Autodesk Fusion 360 part; units mm, degrees
sketch "Sketch1" plane through (0, 0, 0) normal (0, 0, 1) x (1, 0, 0)
  line L0 (17, -17) -> (-17, -17) construction
  line L1 (-17, -17) -> (-17, 17) construction
  line L2 (-17, 17) -> (17, 17) construction
  line L3 (17, 17) -> (17, -17) construction
  line L4 (17, -17) -> (-17, 17) construction
  line L5 (-17, -17) -> (17, 17) construction
  circle A0 centre (17, -17) radius 3
  circle A1 centre (17, 17) radius 3
  circle A2 centre (-17, 17) radius 3
  circle A3 centre (-17, -17) radius 3
  line L6 (-19, -9.5) -> (19, -9.5) construction
  circle A4 centre (19, -9.5) radius 1.5
  circle A5 centre (-19, -9.5) radius 1.5
  circle A6 centre (0, 0) radius 26
  dimension "d1" = 34
  dimension "d2" = 34
  dimension "d3" = 6
  dimension "d4" = 6
  dimension "d5" = 6
  dimension "d6" = 6
  dimension "d7" = 38
  dimension "d8" = 7.5
  dimension "d9" = 3
  dimension "d10" = 3
  dimension "d11" = 52
extrude "Extrude1" add sketch "Sketch1" along normal blind 1.6 contours A0 A1 A2 A3 A6
sketch "Sketch2" plane through (0, 0, 1.6) normal (0, 0, 1) x (1, 0, 0)
  circle A0 centre (-19, -9.5) radius 1.5
  circle A1 centre (19, -9.5) radius 1.5
  line L0 (6, 19) -> (6, 15)
  line L1 (-6, 19) -> (6, 19)
  circle A2 centre (8.75, -12) radius 1.25
  line L2 (6, 15) -> (-6, 19) construction
  circle A3 centre (8.75, -12) radius 2.5
  circle A4 centre (-8.75, -12) radius 2.5
  line L3 (-6, 15) -> (6, 19) construction
  line L4 (6, 15) -> (-6, 15)
  line L5 (-6, 15) -> (-6, 19)
  line L6 (-8.75, -12) -> (8.75, -12) construction
  circle A5 centre (-8.75, -12) radius 1.25
  line L7 (0, 30) -> (0, -30) construction
  point P0 (0, 17)
  point P1 (0, -12)
  dimension "d23" = 12
  dimension "d24" = 4
  dimension "d25" = 17.5
  dimension "d26" = 2.5
  dimension "d27" = 5
  dimension "d28" = 5
  dimension "d29" = 2.5
extrude "Extrude2" add sketch "Sketch2" along normal blind 2 contours L0 L1 L4 L5 | A3 | A4
extrude "Extrude3" cut sketch "Sketch2" against normal blind 2 contours A2 | A5
sketch "Sketch3" plane through (0, 0, 1.6) normal (0, 0, 1) x (1, 0, 0)
  line L0 (-6, 15) -> (-6, 19)
  line L1 (-6, 19) -> (6, 19)
  line L2 (6, 19) -> (6, 15)
  line L3 (6, 15) -> (-6, 15)
  circle A0 centre (8.75, -12) radius 2.5
  circle A1 centre (-19, -9.5) radius 1.5
  circle A2 centre (19, -9.5) radius 1.5
  arc A3 (-16.6394, -19.9782) -> (16.6394, -19.9782) centre (0, 0) ccw
  arc A4 (19.9782, -16.6394) -> (16.6394, -19.9782) centre (17, -17) ccw
  arc A5 (19.9782, -16.6394) -> (19.9782, 16.6394) centre (0, 0) ccw
  arc A6 (16.6394, 19.9782) -> (19.9782, 16.6394) centre (17, 17) ccw
  arc A7 (16.6394, 19.9782) -> (-16.6394, 19.9782) centre (0, 0) ccw
  arc A8 (-19.9782, 16.6394) -> (-16.6394, 19.9782) centre (-17, 17) ccw
  arc A9 (-19.9782, 16.6394) -> (-19.9782, -16.6394) centre (0, 0) ccw
  arc A10 (-16.6394, -19.9782) -> (-19.9782, -16.6394) centre (-17, -17) ccw
  circle A11 centre (-8.75, -12) radius 2.5
  line L4 (-6.375, -20) -> (6.375, -20)
  circle A12 centre (6.375, -20) radius 1.25
  circle A13 centre (-6.375, -20) radius 1.25
  point P0 (0, -20)
  point P1 (8.75, -12)
  dimension "d36" = 12.75
  dimension "d37" = 8
  dimension "d38" = 2.5
  dimension "d39" = 2.5
extrude "Extrude5" cut sketch "Sketch3" against normal through all contours A12 | A13
Build history of the part. All positions in model axes, mm. A direction names the side the tool comes from. Give positions to 0.01 mm unless a question says otherwise; leave off trailing zeros. Loops run counter-clockwise (first coordinate to the right, second up) from the corner with the lowest first, then second, coordinate; pieces in that order, holes last.
Item 1: Drill centre lines: line 1 (X direction, y = -10, z = 0.4); line 2 (Z direction, x = 10.5, y = 14); line 3 (Y direction, x = 17, z = 0.8). Where is each one in solid material? Low to high.
Answers follow:
line 1: x = -24 to -20.41, -17.59 to 17.59, 20.41 to 24
line 2: z = 0 to 1.6
line 3: y = -14 to 14
Item 2: Slice it at A-A, the plane z = 3.05. List the corners of the cut face in (x, y), and give its area (3 significant figures).
Answers follow:
outline: circle Ø5 at (-8.75, -12); (-6, 15) - (6, 15) - (6, 19) - (-6, 19) - close; circle Ø5 at (8.75, -12); hole circle Ø2.5 at (-8.75, -12); hole circle Ø2.5 at (8.75, -12)
area: 77.5 mm2
Item 3: Slice it at C-C, the plane x = -19. List the corners of the cut face in (y, z).
Answers follow:
outline: (-14.76, 0) - (-11, 0) - (-11, 1.6) - (-14.76, 1.6) - close; (-8, 0) - (14.76, 0) - (14.76, 1.6) - (-8, 1.6) - close
Item 4: Slice it at B-B, the plane y = -12. List the corners of the cut face in (x, z), and give its area (3 significant figures).
Answers follow:
outline: (-23.07, 0) - (-10, 0) - (-10, 3.6) - (-11.25, 3.6) - (-11.25, 1.6) - (-23.07, 1.6) - close; (-7.5, 0) - (7.5, 0) - (7.5, 3.6) - (6.25, 3.6) - (6.25, 1.6) - (-6.25, 1.6) - (-6.25, 3.6) - (-7.5, 3.6) - close; (10, 0) - (23.07, 0) - (23.07, 1.6) - (11.25, 1.6) - (11.25, 3.6) - (10, 3.6) - close
area: 75.8 mm2
Item 5: Which spindle directions (+Z, -Z, +X, -X, +Y, -Y) get a long thin tool onto all of the face, cutting with end or side? Do faces 4 (the face through (8.21, -9.56, 2.59)), 5 (the face through (0, 19, 3)), 6 (the face through (-6, 17, 3)). Say none if no direction does.
Answers follow:
face 4: +Z
face 5: +Z, +X, -X, +Y
face 6: +Z, -X, +Y, -Y
Item 6: Flat gauge pins, fed straight in: pin 1 (1 mm diameter, centred on y = 17, z = 3, fed in from +X); pin 2 (10 mm diameter, centred on x = 18, y = 13, fed in from +Z); pin 3 (0.6 mm diameter, centred on x = -2.5, z = 2.5, fed in from -Y). Where does each tip first touch, or does it go through?
Answers follow:
pin 1: stops at x = 6
pin 2: stops at z = 1.6
pin 3: stops at y = 15
Item 7: Slice it at D-D, the plane x = 1. List the corners of the cut face in (y, z), and give its area (3 significant figures).
Answers follow:
outline: (-25.98, 0) - (25.98, 0) - (25.98, 1.6) - (19, 1.6) - (19, 3.6) - (15, 3.6) - (15, 1.6) - (-25.98, 1.6) - close
area: 91.1 mm2
Item 8: Pull direction Y, two halves, no side cores. Call faces 1 (the face through (0, 26, 1)), 2 (the face through (-6.65, -21.22, 0.81)), 3 (the face through (0, 0, 0)): released by +Y, released by -Y, zero draft, split by the parting line, or undercut.
Answers follow:
face 1: released by +Y
face 2: undercut
face 3: zero draft
